The listing builds one solid part. Answer for the finished solid, in the listing's coordinates (mm). Face numbers are marked on the shaded views. A direction names the side the tool comes from. Round coordinates to 2 decimals unless told otherwise and drop trailing zeros. Order: outer loops, then holes, each group sorted by start corner. A loop starts at its lowest first (then second) coordinate and runs counter-clockwise, first axis right, second up. Notation, with made-up numbers: M -13,51 L 17,51 A33 cw 17,83 Z; hole C 53.25,-19 d6. An arc over 180 degrees is marked long. Write item = value, one per line. Start each with the question number.
(1) For a pull along Z with two mould halves and no side action, classify the marked faces 1, 2 and 3 as released by +Z, released by -Z, zero draft, split by the parting line, or undercut.
(2) Straight lines are drawn through the part: probe 1 along X at (y, z) = (10, 45.5); probe 2 along X at (y, z) = (3.5, 62.75); probe 3 along Z at (x, y) = (-100, 6.75). For each, find the intervals that lie inside material, in ascending order. Write a range as from..to.
(3) Each of these flat-tipped pins is pushed along its axis until it touches: pin 1 (3 mm diameter, centred on x = -14, y = 11.5, fed in from -Z); pin 2 (11 mm diameter, centred on x = -75.5, y = 11.5, fed in from -Z); pin 3 (9 mm diameter, centred on x = -99.5, z = 55.5, fed in from -Y). Where does it stop, or does it pass through?
(4) A cutting plane is placed at C-C, the plane y = 13.5. Determine the outline of the cut face in (x, z).
(5) A cutting plane is placed at A-A, the plane z = 9.5. Determine the outline of the cut face in (x, y), and give its area (3 significant figures).
(6) A cutting plane is placed at B-B, the plane x = -15. Determine the outline of the cut face in (y, z).
(7) Which of the six approach directions +Z, -Z, +X, -X, +Y, -Y give full straight-line access (tool end or side, diameter ignored) to the marked faces 4 and 5?
(8) A cutting plane is placed at D-D, the plane z = 62.75. Determine the outline of the cut face in (x, y).
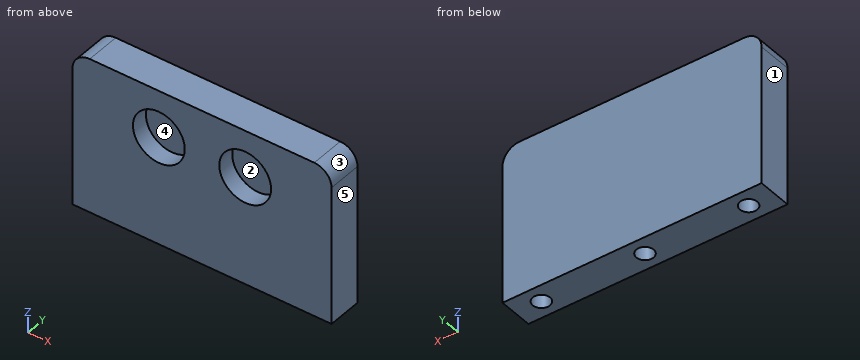
from build123d import *

# Parameters (mm, degrees)
SKETCH1_W               = 90
SKETCH1_H               = 20
BOSS_EXTRUDE1_DEPTH     = 150
CUT_EXTRUDE1_DEPTH      = 177.068168617
CUT_EXTRUDE1_DEPTH_BACK = 10
SKETCH2_R               = 15
CUT_EXTRUDE3_DEPTH      = 177.068168617
CUT_EXTRUDE3_DEPTH_BACK = 70
SKETCH4_R               = 5
FILLET1_R               = 10


with BuildPart() as part:
    # Sketch1 → Boss-Extrude1 (new body)
    with BuildSketch(Plane(origin=(0, 0, 0), x_dir=(0, 0, -1), z_dir=(1, 0, 0))):
        with Locations((-45, 10)):
            Rectangle(SKETCH1_W, SKETCH1_H)
    extrude(amount=-BOSS_EXTRUDE1_DEPTH)

    # Sketch2 → Cut-Extrude1 (cut, two sides: drawn at the far end of the back side and taken through both)
    with BuildSketch(Plane.XZ.offset(-CUT_EXTRUDE1_DEPTH_BACK)):
        with Locations(Location((-50, 62.75, 0), (0, 0, 90))):
            Circle(SKETCH2_R)
        with Locations(Location((-100, 62.75, 0), (0, 0, 90))):
            Circle(SKETCH2_R)
    extrude(amount=CUT_EXTRUDE1_DEPTH + CUT_EXTRUDE1_DEPTH_BACK, mode=Mode.SUBTRACT)

    # Sketch4 → Cut-Extrude3 (cut, two sides: drawn at the far end of the back side and taken through both)
    with BuildSketch(Plane(origin=(0, 0, 0), x_dir=(-1, 0, 0), z_dir=(0, 0, -1)).offset(-CUT_EXTRUDE3_DEPTH_BACK)):
        with Locations(Location((15, 10, 0), (0, 0, 180))):
            Circle(SKETCH4_R)
        with Locations(Location((75, 10, 0), (0, 0, 180))):
            Circle(SKETCH4_R)
        with Locations(Location((135, 10, 0), (0, 0, 180))):
            Circle(SKETCH4_R)
    extrude(amount=CUT_EXTRUDE3_DEPTH + CUT_EXTRUDE3_DEPTH_BACK, mode=Mode.SUBTRACT)

    # Fillet1
    fillet1_edges = [part.edges().sort_by_distance(p)[0] for p in [
        (-150, 10, 90),
        (0, 10, 90),
    ]]
    fillet(fillet1_edges, radius=FILLET1_R)


solid = part.part
Reported:
q1.face_1 = zero draft
q1.face_2 = undercut
q1.face_3 = released by +Z
q2.probe_1 = -150..-140, -130..-80, -70..-20, -10..0
q2.probe_2 = -150..-115, -85..-65, -35..0
q2.probe_3 = 0..47.75, 77.75..90
q3.pin_1 = 70
q3.pin_2 = 0
q3.pin_3 = 10
q4.outline = M -150,0 L -138.57,0 L -138.57,70 L -131.43,70 L -131.43,0 L -78.57,0 L -78.57,70 L -71.43,70 L -71.43,0 L -18.57,0 L -18.57,70 L -11.43,70 L -11.43,0 L 0,0 L 0,80 A10 ccw -10,90 L -140,90 A10 ccw -150,80 Z
q5.outline = M -150,0 L 0,0 L 0,20 L -150,20 Z; hole C -135,10 d10; hole C -75,10 d10; hole C -15,10 d10
q5.area = 2,760 mm²
q6.outline = M 0,0 L 5,0 L 5,70 L 15,70 L 15,0 L 20,0 L 20,90 L 0,90 Z
q7.face_4 = -Y
q7.face_5 = +Z, -Z, +X, +Y, -Y
q8.outline = M -150,0 L -115,0 L -115,10 L -85,10 L -85,0 L -65,0 L -65,10 L -35,10 L -35,0 L 0,0 L 0,20 L -150,20 Z; hole C -135,10 d10; hole C -75,10 d10; hole C -15,10 d10
